Job drawing, mm, ordinate dimensions from the low corner. One solid piece. A direction names the side the tool comes from. Round coordinates to 2 decimals unless told otherwise and drop trailing zeros. Loops run counter-clockwise (first coordinate to the right, second up) from the corner with the lowest first, then second, coordinate; pieces in that order, holes last.
1) 3-axis set-ups, long thin cutter, end or side, ignore diameter. For the marked faces 4, 5 and 6: which of +Z, -Z, +X, -X, +Y, -Y reach the whole face in a straight line?
2) Band-saw the part on D-D, the plane y = 31.5. Write the cut outline in (x, z), then the cut area to 3 significant figures.
3) Band-saw the part on A-A, the plane y = 19.5. Write the cut outline in (x, z) (1 decimal).
4) Band-saw the part on B-B, the plane x = 19. Write the cut outline in (y, z).
5) Probe line 1 (X direction, y = 10, z = 25); line 2 (Z direction, x = 57, y = 8); line 3 (Y direction, x = 18, z = 18.5). List the from-to ranges inside material, lowest first.
6) Mould opens along Z. For the marked faces 1, 2 and 3 say: +Z half, -Z half, draft (parallel to the pull), parting line (faces both ways), or undercut.
7) Band-saw the part on C-C, the plane z = 20.5. Write the cut outline in (x, y), then the cut area to 3 significant figures.
8) Drop flat-ended pins along their axis: P1, Ø12, axis at x = 29, z = 41, coming from the +Y side; P2, Ø7.5, axis at y = 21.5, z = 9, coming from the -X side; P3, Ø5, axis at x = 49.5, y = 25.5, coming from the +Z side. Give the stop position or say it passes through.
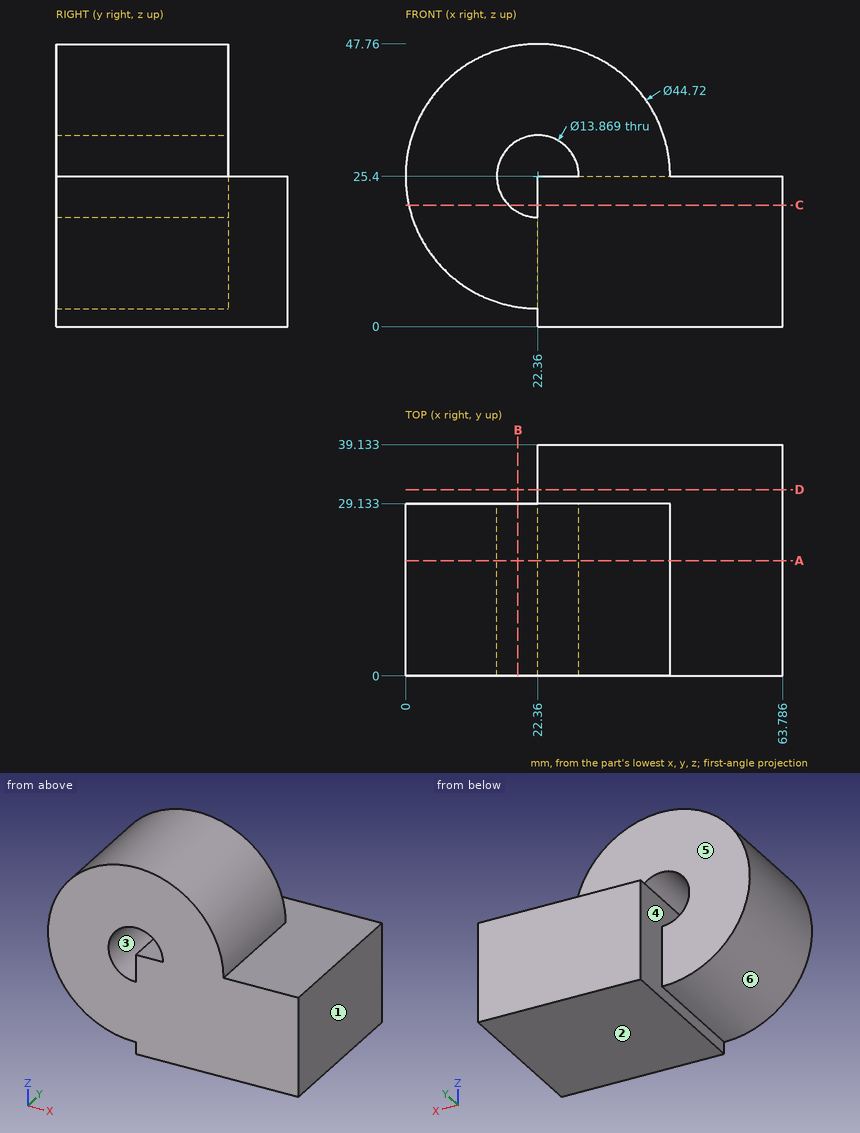
Reported:
1. face 4: +Y
1. face 5: +Z, -X, +Y
1. face 6: +Y, -Y
2. outline: (22.36, 0) - (63.79, 0) - (63.79, 25.4) - (22.36, 25.4) - close
2. area: 1,050 mm2
3. outline: (22.4, 0) - (63.8, 0) - (63.8, 25.4) - (44.7, 25.4) arc R22.4 ccw (long way) to (22.4, 3) - close; hole (22.4, 18.5) - (22.4, 25.4) - (29.3, 25.4) arc R6.9 ccw (long way) to start
4. outline: (0, 3.29) - (29.13, 3.29) - (29.13, 19.33) - (0, 19.33) - close; (0, 31.47) - (29.13, 31.47) - (29.13, 47.51) - (0, 47.51) - close
5. line 1: x = 0 to 15.44, 22.36 to 63.79
5. line 2: z = 0 to 25.4
5. line 3: y = 0 to 29.13
6. face 1: draft
6. face 2: -Z half
6. face 3: undercut
7. outline: (0.54, 0) - (17.45, 0) - (17.45, 29.13) - (0.54, 29.13) - close; (22.36, 0) - (63.79, 0) - (63.79, 39.13) - (22.36, 39.13) - close
7. area: 2,110 mm2
8. P1: stops at y = 29.13
8. P2: stops at x = 3.92
8. P3: stops at z = 25.4
